Geometry check sheet. Reference: drawing and pictorial views, mm from the part's lowest x, y, z. A direction names the side the tool comes from. Round coordinates to 2 decimals unless told otherwise and drop trailing zeros. Write each loop counter-clockwise with the first axis right and the second up, starting at its lowest first coordinate (ties: lowest second). Pieces come first, ordered by that corner, then holes. Notation, with made-up numbers: (58, -15.75) -> (114, -15.75) arc R20 ccw to (114, 2.25) -> close; hole circle Ø3 at (-4.75, 75). An arc over 180 degrees is marked (long way). Write item = value, one per line.
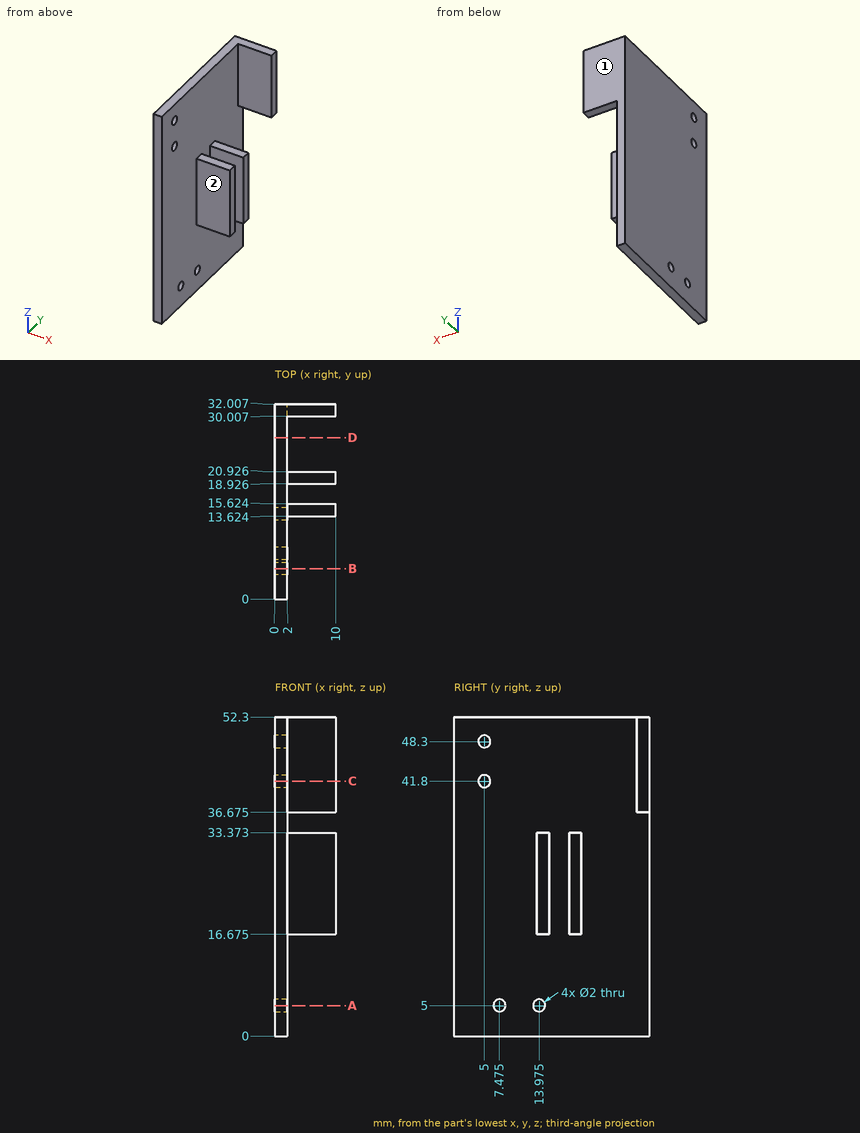
(1) Go/stop test with flat-tipped pins: P1, Ø1, axis at y = 5.5, z = 34, coming from the +X side; P2, Ø2.5, axis at x = 5.5, z = 26.5, coming from the +Y side; P3, Ø1.6, axis at x = 5.5, y = 14.5, coming from the +Z side; P4, Ø1.6, axis at y = 7.47, z = 5, coming from the +X side. Record where each tip stops, or that it passes through.
Worked answers:
P1 = 2
P2 = 20.93
P3 = 33.37
P4 = through
(2) Sectioned sample at A-A on z = 5. Enter the section's corners in (x, y) (3 decimals), then the cut area to 3 significant figures.
Worked answers:
outline = (0, 0) -> (2, 0) -> (2, 6.475) -> (0, 6.475) -> close; (0, 8.475) -> (2, 8.475) -> (2, 12.975) -> (0, 12.975) -> close; (0, 14.975) -> (2, 14.975) -> (2, 32.007) -> (0, 32.007) -> close
area = 56.0 mm²
(3) Access from +Z, -Z, +X, -X, +Y, -Y to the whole of each face (thin tool, end or side, straight path). Record for the marked faces 1 and 2.
Worked answers:
face_1 = +Z, -Z, +X, -X, +Y
face_2 = +Z, -Z, +X, -Y
(4) Sectioned sample at C-C on z = 41.8. Enter the section's corners in (x, y).
Worked answers:
outline = (0, 0) -> (2, 0) -> (2, 4) -> (0, 4) -> close; (0, 6) -> (2, 6) -> (2, 30.01) -> (10, 30.01) -> (10, 32.01) -> (0, 32.01) -> close
(5) Sectioned sample at B-B on y = 5. Enter the section's corners in (x, z).
Worked answers:
outline = (0, 0) -> (2, 0) -> (2, 40.8) -> (0, 40.8) -> close; (0, 42.8) -> (2, 42.8) -> (2, 47.3) -> (0, 47.3) -> close; (0, 49.3) -> (2, 49.3) -> (2, 52.3) -> (0, 52.3) -> close
(6) Sectioned sample at D-D on y = 26.5. Enter the section's corners in (x, z).
Worked answers:
outline = (0, 0) -> (2, 0) -> (2, 52.3) -> (0, 52.3) -> close
(7) Material ranges on L1, parallel to Y at x = 1.4, z = 5 (3 decimals); L2, parallel to Z at x = 1.25, y = 5; L3, parallel to Y at x = 9.5, z = 25, recorded low to high. Write a range as [from, to].
Worked answers:
L1 = [0, 6.475], [8.475, 12.975], [14.975, 32.007]
L2 = [0, 40.8], [42.8, 47.3], [49.3, 52.3]
L3 = [13.62, 15.62], [18.93, 20.93]
